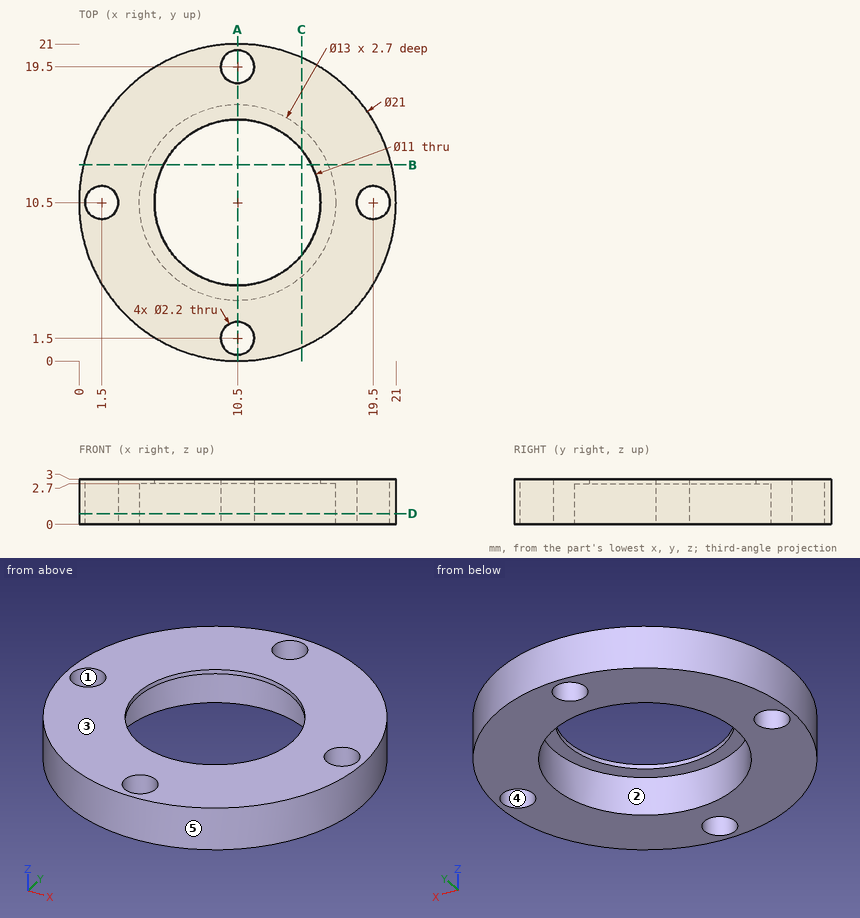
The figure shows three views and two pictorial views of one solid part (mm, origin at its lowest corner). Answer the questions. A direction names the side the tool comes from. Coordinates: 2 decimals unless noted, no trailing zeros. Loops run counter-clockwise (first coordinate to the right, second up) from the corner with the lowest first, then second, coordinate; pieces in that order, holes last. Notation, with made-up numbers: M -39.5,-29 L -1.5,-29 A28 cw -1.5,-7 Z; hole C 44,21.25 d10. An arc over 180 degrees is marked long. Use CSV: the item, a comma, the result in double quotes. Start each with the question number.
(1) For a pull along Y with two mould halves and no side action, classify the marked faces 3, 4 and 5 as +Y half, -Y half, draft (parallel to the pull), parting line (faces both ways), or undercut.
(2) For the marked faces 1 and 2, determine the directions among +Z, -Z, +X, -X, +Y, -Y from which every point of the face is accessible in a straight line to the end or side of a thin tool.
(3) Find section B-B, the plane y = 13. Give the vertices of the cut face in (x, z), then the cut area to 3 significant figures.
(4) Find section D-D, the plane z = 0.7. Give the vertices of the cut face in (x, y), then the cut area to 3 significant figures.
(5) Given pin 1 Ø11.5 at (x, y) = (10.5, 10.5) entering from -Z; pin 2 Ø12.5 at (x, y) = (10.5, 10.5) entering from +Z; pin 3 Ø1.5 at (y, z) = (12.5, 1.5) entering from -X, each flat-ended and moving along its own axis, determine where each tip first touches the part or whether it passes through.
(6) Find section C-C, the plane x = 14.75. Give the vertices of the cut face in (y, z), then the cut area to 3 significant figures.
(7) Consider line 1 (Y direction, x = 10.5, z = 1.3); line 2 (Y direction, x = 11.5, z = 1.6); line 3 (X direction, y = 2.25, z = 1.15). Determine where each line is inside the solid, lowest interval first.
(8) Find section A-A, the plane x = 10.5. Give the vertices of the cut face in (y, z).
Recorded:
1,face 3,"draft"
1,face 4,"undercut"
1,face 5,"parting line"
2,face 1,"+Z, -Z"
2,face 2,"-Z"
3,outline,"M 0.3,0 L 4.5,0 L 4.5,2.7 L 5.6,2.7 L 5.6,3 L 0.3,3 Z; M 15.4,2.7 L 16.5,2.7 L 16.5,0 L 20.7,0 L 20.7,3 L 15.4,3 Z"
3,area,"25.8 mm^2"
4,outline,"C 10.5,10.5 d21; hole C 1.5,10.5 d2.2; hole C 10.5,10.5 d13; hole C 10.5,1.5 d2.2; hole C 10.5,19.5 d2.2; hole C 19.5,10.5 d2.2"
4,area,"198 mm^2"
5,pin 1,"stops at z = 2.7"
5,pin 2,"stops at z = 3"
5,pin 3,"stops at x = 0.07"
6,outline,"M 0.9,0 L 5.58,0 L 5.58,2.7 L 7.01,2.7 L 7.01,3 L 0.9,3 Z; M 13.99,2.7 L 15.42,2.7 L 15.42,0 L 20.1,0 L 20.1,3 L 13.99,3 Z"
6,area,"29.0 mm^2"
7,line 1,"y = 0 to 0.4, 2.6 to 4, 17 to 18.4, 20.6 to 21"
7,line 2,"y = 0.05 to 1.04, 1.96 to 4.08, 16.92 to 19.04, 19.96 to 20.95"
7,line 3,"x = 4 to 9.7, 11.3 to 17"
8,outline,"M 0,0 L 0.4,0 L 0.4,3 L 0,3 Z; M 2.6,0 L 4,0 L 4,2.7 L 5,2.7 L 5,3 L 2.6,3 Z; M 16,2.7 L 17,2.7 L 17,0 L 18.4,0 L 18.4,3 L 16,3 Z; M 20.6,0 L 21,0 L 21,3 L 20.6,3 Z"
